Design review of the part built by this model. Coordinates are the model's own, in mm. A direction names the side the tool comes from. Round coordinates to 2 decimals unless told otherwise and drop trailing zeros. Order: outer loops, then holes, each group sorted by start corner. A loop starts at its lowest first (then second) coordinate and runs counter-clockwise, first axis right, second up. Notation, with made-up numbers: M -17,43 L 18,43 A23 cw 18,58 Z; hole C -7,-1.75 d2. An arc over 180 degrees is marked long. Write item = value, one per line. Start each with the question number.
Autodesk Inventor part; units mm, degrees
ref_plane "FDT_ANBAU_XY" through (0, 0, -1.5) normal (0, 0, -1) x (1, 0, 0)
ref_plane "FDT_ANBAU_YZ" through (0, 0, -1.5) normal (1, 0, 0) x (0, -1, 0)
ref_plane "FDT_ANBAU_ZX" through (0, 0, -1.5) normal (0, -1, 0) x (0, 0, -1)
sketch "Skizze_1" plane through (0, 0, 0) normal (1, 0, 0) x (0, 1, 0)
  line L0 (0, -52.05) -> (0, 0)
  line L1 (0, -7) -> (3.1, -7)
  line L2 (3.1, -7) -> (3.1, 0)
  line L3 (3.1, 0) -> (4.3865, 0)
  line L4 (4.3865, 0) -> (5, -0.6135)
  line L5 (5, -0.6135) -> (5, -40.4365)
  line L6 (5, -40.4365) -> (4.3865, -41.05)
  line L7 (4.3865, -41.05) -> (4.3, -41.05)
  line L8 (4.3, -41.05) -> (4.3, -51.55)
  line L9 (4.3, -51.55) -> (3.8, -52.05)
  line L10 (3.8, -52.05) -> (0, -52.05)
  line L11 (0, -52.05) -> (0, -7)
revolve "Revolution1" add sketch "Skizze_1" angle 360 about axis through (0, 0, -52.05) along (0, 0, -1)
thread "Thread1"
sketch "Skizze_3" plane through (0, 0, 0) normal (1, 0, 0) x (0, 1, 0)
  line L0 (0, -14) -> (0, 10)
  arc A0 (3, 9.8118) -> (0, 10) centre (0, -14) ccw
  line L1 (3, 9.8118) -> (3, 3)
  line L2 (3, 3) -> (1.5, 3)
  line L3 (1.5, 3) -> (1.5, -14)
  line L4 (1.5, -14) -> (0, -14)
  line L5 (0, -14) -> (0, 10)
revolve "Revolution2" add sketch "Skizze_3" angle 360 about axis through (0, 0, -14) along (0, 0, -1)
sketch "Skizze_4" plane through (0, 0, -52.05) normal (0, 0, -1) x (0, 1, 0)
  line L0 (-1.5, -0.866) -> (0, -1.7321)
  line L1 (0, -1.7321) -> (1.5, -0.866)
  line L2 (1.5, -0.866) -> (1.5, 0.866)
  line L3 (1.5, 0.866) -> (0, 1.7321)
  line L4 (0, 1.7321) -> (-1.5, 0.866)
  line L5 (-1.5, 0.866) -> (-1.5, -0.866)
extrude "Extrusion1" cut sketch "Skizze_4" against normal blind 2
ref_plane "FDT_ANBAU_XY" through (0, 0, -1.5) normal (0, 0, -1) x (1, 0, 0)
ref_plane "FDT_ANBAU_YZ" through (0, 0, -1.5) normal (1, 0, 0) x (0, -1, 0)
ref_plane "FDT_ANBAU_ZX" through (0, 0, -1.5) normal (0, -1, 0) x (0, 0, -1)
ref_plane "FDT_NUT_XY" through (0, 0, -21.5) normal (0, 0, 1) x (1, 0, 0)
ref_plane "FDT_NUT_YZ" through (0, 0, -21.5) normal (1, 0, 0) x (0, 1, 0)
ref_plane "FDT_NUT_ZX" through (0, 0, -21.5) normal (0, 1, 0) x (0, 0, 1)
ref_plane "IP_DGSL_XY" through (0, 0, -52.05) normal (0, 0, -1) x (0, 1, 0)
ref_plane "IP_DGSL_YZ" through (0, 0, -52.05) normal (0, 1, 0) x (1, 0, 0)
ref_plane "IP_DGSL_ZX" through (0, 0, -52.05) normal (1, 0, 0) x (0, 0, -1)
ref_plane "NUT1_XY" through (0, 0, -17.025) normal (0, 0, 1) x (1, 0, 0)
ref_plane "NUT1_YZ" through (0, 0, -17.025) normal (1, 0, 0) x (0, 1, 0)
ref_plane "NUT1_ZX" through (0, 0, -17.025) normal (0, 1, 0) x (0, 0, 1)
ref_plane "NUT2_XY" through (0, 0, -24.025) normal (0, 0, 1) x (1, 0, 0)
ref_plane "NUT2_YZ" through (0, 0, -24.025) normal (1, 0, 0) x (0, 1, 0)
ref_plane "NUT2_ZX" through (0, 0, -24.025) normal (0, 1, 0) x (0, 0, 1)
properties part number "548072 DYSW-7-10-Y1F---(SD_0)"
(1) Insertion check: pin 1 (1 mm diameter, centred on x = 1.5, y = 2.5, fed in from +Z); pin 2 (1.9 mm diameter, centred on x = 0.5, z = -50.5, fed in from +Y); pin 3 (1.9 mm diameter, centred on x = 0, z = -51, fed in from -Y). Each pin has a flat end and moves straight along its axis. Give the tip position at first contact, or say it passes through.
(2) Consider section A-A, the plane z = -4. Write out the cut boundary in (x, y), then the cut area to 3 significant figures.
(3) Draft analysis for pull direction Y (two halves, no side actions). For faces 5 (the face through (-1.3, 1.3, 3)), 6 (the face through (-1.293, -0.76, -51.064)), 7 (the face through (0.189, -4.296, -46.374)), state which applies: pulls with the +Y half, pulls with the -Y half, needs draft (parallel to the pull), parting line crosses it, or undercut.
(4) Consider section B-B, the plane z = -23. Write out the cut boundary in (x, y).
(5) For faces 1 (the face through (0, -3, 6)), 2 (the face through (0.07, -1.5, -2.07)), 3 (the face through (0, -1.5, -51)), 4 (the face through (-4.88, -1.08, -20.8)), list the 3-axis set-ups (+Z, -Z, +X, -X, +Y, -Y) from which the entire face can be reached by the end or side of a thin tool; tool diameter is ignored.
(6) For line 1 along X through (y, z) = (0, -5.5); line 2 along Y through (x, z) = (0.75, -0.5); line 3 along Y through (x, z) = (1, -1.5), list the stretches that pass through material, from the lowest coordinate up. Write a range as [from, to].
Completed:
q1.pin_1 = 9.88
q1.pin_2 = 4.3
q1.pin_3 = -4.3
q2.outline = C 0,0 d10; C 0,0 d3; hole C 0,0 d6.2
q2.area = 55.4 mm2
q3.face_5 = needs draft
q3.face_6 = undercut
q3.face_7 = parting line crosses it
q4.outline = C 0,0 d10
q5.face_1 = +Z
q5.face_2 = none
q5.face_3 = -Z
q5.face_4 = +Z, -Z
q6.line_1 = [-5, -3.1], [-1.5, 1.5], [3.1, 5]
q6.line_2 = [-4.83, -3.01], [-1.3, 1.3], [3.01, 4.83]
q6.line_3 = [-4.9, -2.93], [-1.12, 1.12], [2.93, 4.9]
